Autodesk Inventor part; units mm, degrees
ref_plane "YZ Plane" through (0, 0, 0) normal (1, 0, 0) x (0, 1, 0)
ref_plane "XZ Plane" through (0, 0, 0) normal (0, 1, 0) x (-1, 0, 0)
ref_plane "XY Plane" through (0, 0, 0) normal (0, 0, 1) x (1, 0, 0)
sketch "Sketch1" plane through (0, 0, 0) normal (0, 0, 1) x (1, 0, 0)
  line L0 (-79.5, -92) -> (79.5, -92)
  line L1 (79.5, -92) -> (79.5, 92)
  line L2 (79.5, 92) -> (-79.5, 92)
  line L3 (-79.5, 92) -> (-79.5, -92)
  line L4 (-79.5, -92) -> (79.5, 92) construction
  line L5 (79.5, -92) -> (-79.5, 92) construction
  point P0 (0, 0)
  dimension "d0" = 159
  dimension "d1" = 184
extrude "Extrusion1" add sketch "Sketch1" along normal blind 46
sketch "Sketch2" plane through (0, 0, 46) normal (0, 0, 1) x (1, 0, 0)
  line L0 (-79.5, 92) -> (-79.5, -92)
  line L1 (79.5, -92) -> (79.5, 92)
  line L2 (-79.5, 92) -> (-99.5, 92)
  line L3 (-99.5, 92) -> (-99.5, -92)
  line L4 (-99.5, -92) -> (-79.5, -92)
  line L5 (79.5, -92) -> (99.5, -92)
  line L6 (99.5, -92) -> (99.5, 92)
  line L7 (99.5, 92) -> (79.5, 92)
  point P0 (0, 0)
  dimension "d4" = 20
extrude "Extrusion2" add sketch "Sketch2" against normal blind 5
sketch "Sketch3" plane through (-79.5, 92, 0) normal (0, 1, 0) x (1, 0, 0)
  line L0 (18.6001, -13.4734) -> (39.6187, -13.4734)
  line L1 (39.6187, -13.4734) -> (39.6187, -29.911)
  line L2 (39.6187, -29.911) -> (18.6001, -29.911)
  line L3 (18.6001, -29.911) -> (18.6001, -13.4734)
  line L4 (54.4394, -15.0902) -> (73.3022, -15.0902)
  line L5 (73.3022, -15.0902) -> (73.3022, -29.911)
  line L6 (73.3022, -29.911) -> (54.4394, -29.911)
  line L7 (54.4394, -29.911) -> (54.4394, -15.0902)
  line L8 (94.5902, -13.4734) -> (112.9141, -13.4734)
  line L9 (112.9141, -13.4734) -> (112.9141, -28.5637)
  line L10 (112.9141, -28.5637) -> (94.5902, -28.5637)
  line L11 (94.5902, -28.5637) -> (94.5902, -13.4734)
  line L12 (131.5074, -13.4734) -> (153.3344, -13.4734)
  line L13 (153.3344, -13.4734) -> (153.3344, -28.5637)
  line L14 (153.3344, -28.5637) -> (131.5074, -28.5637)
  line L15 (131.5074, -28.5637) -> (131.5074, -13.4734)
  point P0 (79.5, 0)
extrude "Extrusion3" cut sketch "Sketch3" against normal blind 25.4
sketch "Sketch4" plane through (0, 0, 46) normal (0, 0, 1) x (1, 0, 0)
  circle A0 centre (-93.5, 79) radius 4
  circle A1 centre (93.5, 79) radius 4
  circle A2 centre (93.5, -57) radius 4
  circle A3 centre (-93.5, -57) radius 4
  line L0 (-99.5, 92) -> (99.5, 92)
  line L1 (-99.5, -92) -> (-99.5, 92)
  line L2 (99.5, 92) -> (99.5, -92)
  line L3 (93.5, 79) -> (-93.5, 79) construction
  line L4 (93.5, 79) -> (93.5, -57) construction
  line L5 (-93.5, -57) -> (-93.5, 79) construction
  line L6 (-99.5, 92) -> (-93.5, 79) construction
  line L7 (93.5, 79) -> (99.5, 92) construction
  line L8 (79.5, 92) -> (79.5, -92)
  line L9 (-79.5, -92) -> (-79.5, 92)
  line L10 (79.5, 69) -> (99.5, 69)
  line L11 (79.5, -47) -> (99.5, -47)
  line L12 (79.5, -67) -> (99.5, -67)
  line L13 (99.5, -92) -> (79.5, -92)
  line L14 (-79.5, -92) -> (-99.5, -92)
  line L15 (-79.5, -67) -> (-99.5, -67)
  line L16 (-79.5, -47) -> (-99.5, -47)
  line L17 (-79.5, 69) -> (-99.5, 69)
  line L18 (79.5, 89) -> (99.5, 89)
  line L19 (-99.5, 89) -> (-79.5, 89)
  point P0 (0, 0)
  dimension "d9" = 13
  dimension "d10" = 8
  dimension "d11" = 149
  dimension "d12" = 187
  dimension "d13" = 23
  dimension "d14" = 139
  dimension "d15" = 159
  dimension "d22" = 3
extrude "Extrusion4" cut sketch "Sketch4" against normal up to surface (5 mm away) contours A0 | A1 | A2 | A3 | L0 L2 L18 L8 | L0 L9 L19 L1 | L17 L9 L16 L1 | L10 L2 L11 L8 | L15 L9 L14 L1 | L12 L2 L13 L8
sketch "Sketch5" plane through (0, 0, 41) normal (0, 0, -1) x (-1, 0, 0)
  circle A0 centre (-93.5, 79) radius 4
  line L0 (-79.5, 89) -> (-79.5, 69)
  line L1 (-99.5, 69) -> (-79.5, 69)
  line L2 (-79.5, -47) -> (-99.5, -47)
  line L3 (-79.5, -47) -> (-79.5, -67)
  line L4 (-99.5, -67) -> (-79.5, -67)
  circle A1 centre (-93.5, -57) radius 4
  line L5 (-79.5, 89) -> (-99.5, 89)
  line L6 (-93.5, 89) -> (-93.5, 69) construction
  arc A2 (-93.5, 69) -> (-93.5, 89) centre (-93.5, 79) ccw
  line L7 (-93.5, -47) -> (-93.5, -67) construction
  arc A3 (-93.5, -67) -> (-93.5, -47) centre (-93.5, -57) ccw
  point P0 (0, 0)
extrude "Extrusion5" add sketch "Sketch5" along normal blind 25.4 contours L0 L1 A2 L5 | L3 L4 A3 L2
properties part number "MCM"
Input: part model. Units: mm. Frame: model coordinates. A direction names the side the tool comes from. Round coordinates to 2 decimals unless told otherwise and drop trailing zeros. Loops run counter-clockwise (first coordinate to the right, second up) from the corner with the lowest first, then second, coordinate; pieces in that order, holes last. Notation, with made-up numbers: (-7, -9) -> (-2, -9) arc R25 cw to (-2, 26) -> close; hole circle Ø9 at (73.25, -15.5). An arc over 180 degrees is marked (long way). Use one line per item in the form item = value. Start each with the question number.
Item 1: Material intervals for L1, parallel to Y at x = -93, z = 44; L2, parallel to Y at x = -86.5, z = 42.5; L3, parallel to X at y = -9.5, z = 33.5, sorted ascending. Write a range as from..to.
Item 2: Section query B-B on x = 87. Return the cut outline in (y, z).
Item 3: Set-up query: faces 4 (the face through (-39.881, 79, 22)), 5 (the face through (87, -67, 31)), 6 (the face through (83.5, -56.8, 28.5)). Return all of +Z, -Z, +X, -X, +Y, -Y with unobstructed straight access to the full face (end or side cutting, diameter ignored); none if empty.
Item 4: Mould query, pull axis X, two halves, no side actions, for faces 1 (the face through (-99.5, -57, 44)), 2 (the face through (92.633, -60.905, 43.535)), 3 (the face through (-1, 1, 46)). Classes: pulls with the +X half, pulls with the -X half, needs draft (parallel to the pull), parting line crosses it, or undercut.
Item 5: Section query C-C on x = -12. Return the cut outline in (y, z).
Item 6: Section query D-D on y = 47. Return the cut outline in (x, z).
Item 7: Contact query for flat-ended pins moving along their axis: pin 1 Ø9 at (x, y) = (93.5, 79) entering from -Z; pin 2 Ø6 at (x, z) = (89.5, 26) entering from -Y; pin 3 Ø8 at (x, y) = (87.5, -54) entering from -Z. Output: stop coordinate, or through.
Item 8: Section query A-A on y = -57. Return the cut outline in (x, z), then the cut area to 3 significant figures.
Ans:
q1.L1 = -67..-60.97, -53.03..-47, 69..75.03, 82.97..89
q1.L2 = -67..-47, 69..89
q1.L3 = -79.5..79.5
q2.outline = (-67, 15.6) -> (-64.6, 15.6) -> (-64.6, 41) -> (-49.4, 41) -> (-49.4, 15.6) -> (-47, 15.6) -> (-47, 46) -> (-67, 46) -> close; (69, 15.6) -> (71.4, 15.6) -> (71.4, 41) -> (86.6, 41) -> (86.6, 15.6) -> (89, 15.6) -> (89, 46) -> (69, 46) -> close
q3.face_4 = +Y
q3.face_5 = +Z, -Z, +X, -Y
q3.face_6 = -Z, +X
q4.face_1 = pulls with the -X half
q4.face_2 = undercut
q4.face_3 = needs draft
q5.outline = (-92, 0) -> (92, 0) -> (92, 15.09) -> (66.6, 15.09) -> (66.6, 29.91) -> (92, 29.91) -> (92, 46) -> (-92, 46) -> close
q6.outline = (-79.5, 0) -> (79.5, 0) -> (79.5, 46) -> (-79.5, 46) -> close
q7.pin_1 = 41
q7.pin_2 = -67
q7.pin_3 = 15.6
q8.outline = (-99.5, 41) -> (-97.5, 41) -> (-97.5, 46) -> (-99.5, 46) -> close; (-89.5, 41) -> (-79.5, 41) -> (-79.5, 0) -> (79.5, 0) -> (79.5, 15.6) -> (83.5, 15.6) -> (83.5, 41) -> (89.5, 41) -> (89.5, 46) -> (-89.5, 46) -> close; (97.5, 41) -> (99.5, 41) -> (99.5, 46) -> (97.5, 46) -> close
q8.area = 7,540 mm^2
